Source: CAD feature listing. Evaluate the final solid. Frame: model axes, mm. A direction names the side the tool comes from. Coordinates: 2 decimals unless noted, no trailing zeros. Loops run counter-clockwise (first coordinate to the right, second up) from the corner with the lowest first, then second, coordinate; pieces in that order, holes last. Notation, with made-up numbers: M -13.5,10 L 36.5,10 A16 cw 36.5,17 Z; hole C -0.5,-31 d4. An arc over 180 degrees is marked long. One line per question, with ' | ' between items. Start each with the question number.
1. Access query for faces 4 (the flat face through (1, 20, -46)), 5 (the flat face through (36, -3, -5)), 6 (the flat face through (2, 11, -47)). Directions: +Z, -Z, +X, -X, +Y, -Y. A direction counts if a zero-diameter tool reaches every point of the face in a straight line with its end or side. Return the directions, or none.
2. Section query D-D, the plane y = -1. Output: boundary loops of the cut face in (x, z), and give its area (3 significant figures).
3. Ray query, probe 1 along Z at (x, y) = (68, 11.75); probe 2 along Z at (x, y) = (6, 5); probe 3 along X at (y, z) = (14, -62). Return the intervals inside material, ascending.
4. Section query C-C, the plane z = -58. Output: boundary loops of the cut face in (x, y), and give its area (3 significant figures).
5. Mould query, pull axis Z, two halves, no side actions, for faces 1 (the flat face through (37, 2, -47)), 2 (the flat face through (36, -7, -89)), 3 (the flat face through (37, 7, 0)). Classes: pulls with the +Z half, pulls with the -Z half, needs draft (parallel to the pull), parting line crosses it, or undercut.
6. Pin query (flat end, axial travel): P1, Ø6, axis at x = 48, z = -40, coming from the +Y side; P2, Ø10, axis at x = 16, z = -67, coming from the -Y side. Return the tip coordinate at first contact, or that it passes through.
7. Section query B-B, the plane x = 65.5. Output: boundary loops of the cut face in (y, z), and give its area (3 significant figures).
```python
from build123d import *

# Parameters (mm, degrees)
SKETCH_1_W          = 74
SKETCH_1_H          = 65
EXTRUDE_1_DEPTH     = 20
SKETCH_2_W          = 70
SKETCH_2_H          = 61
CUT_EXTRUDE_1_DEPTH = 18
SKETCH_3_W          = 5
SKETCH_3_H          = 2
CUT_EXTRUDE_2_DEPTH = 18
SKETCH_4_W          = 74
SKETCH_4_H          = 27
EXTRUDE_2_DEPTH     = 20
CUT_EXTRUDE_3_DEPTH = 18
SKETCH_6_W          = 74
SKETCH_6_H          = 5
EXTRUDE_3_DEPTH     = 7
FILLET_1_R          = 2
FILLET_2_R          = 2
FILLET_3_R          = 2
FILLET_5_R          = 1


with BuildPart() as part:
    # 草图1 → 凸台-拉伸1 (new body)
    with BuildSketch(Plane(origin=(0, 0, 0), x_dir=(1, 0, 0), z_dir=(0, 1, 0))):
        with Locations((37, 32.5)):
            Rectangle(SKETCH_1_W, SKETCH_1_H)
    extrude(amount=EXTRUDE_1_DEPTH)

    # 草图2 → 切除-拉伸1 (cut)
    with BuildSketch(Plane(origin=(0, 20, 0), x_dir=(1, 0, 0), z_dir=(0, 1, 0))):
        with Locations((37, 32.5)):
            Rectangle(SKETCH_2_W, SKETCH_2_H)
    extrude(amount=-CUT_EXTRUDE_1_DEPTH, mode=Mode.SUBTRACT)

    # 草图3 → 切除-拉伸2 (cut)
    with BuildSketch(Plane(origin=(0, 20, 0), x_dir=(1, 0, 0), z_dir=(0, 1, 0))):
        with Locations((4.5, 64)):
            Rectangle(SKETCH_3_W, SKETCH_3_H)
    extrude(amount=-CUT_EXTRUDE_2_DEPTH, mode=Mode.SUBTRACT)

    # 草图4 → 凸台-拉伸2 (add)
    with BuildSketch(Plane.XZ):
        with Locations((37, -78.5)):
            Rectangle(SKETCH_4_W, SKETCH_4_H)
    extrude(amount=-EXTRUDE_2_DEPTH)

    # 草图5 → 切除-拉伸3 (cut)
    with BuildSketch(Plane(origin=(0, 20, 0), x_dir=(1, 0, 0), z_dir=(0, 1, 0))):
        Polygon((2, 65), (7, 65), (72, 65), (72, 90), (2, 90), align=None)
    extrude(amount=-CUT_EXTRUDE_3_DEPTH, mode=Mode.SUBTRACT)

    # 草图6 → 凸台-拉伸3 (add)
    with BuildSketch(Plane.XZ):
        with Locations((37, -2.5)):
            Rectangle(SKETCH_6_W, SKETCH_6_H)
        with Locations((37, -89.5)):
            Rectangle(SKETCH_6_W, SKETCH_6_H)
    extrude(amount=EXTRUDE_3_DEPTH)

    # 圆角1
    fillet_1_edges = [part.edges().sort_by_distance(p)[0] for p in [
        (0, 6.5, 0),
    ]]
    fillet(fillet_1_edges, radius=FILLET_1_R)

    # 圆角2
    fillet_2_edges = [part.edges().sort_by_distance(p)[0] for p in [
        (74, 6.5, 0),
    ]]
    fillet(fillet_2_edges, radius=FILLET_2_R)

    # 圆角3
    fillet_3_edges = [part.edges().sort_by_distance(p)[0] for p in [
        (0, 6.5, -92),
        (74, 6.5, -92),
    ]]
    fillet(fillet_3_edges, radius=FILLET_3_R)

    # 圆角5
    fillet_5_edges = [part.edges().sort_by_distance(p)[0] for p in [
        (7, 11, -65),
        (7, 11, -63),
    ]]
    fillet(fillet_5_edges, radius=FILLET_5_R - 0.0001)  # a hair under: the kernel refuses the full size


solid = part.part
```
Taken from the geometry:
1) face 4: +Z, -Z, +X, -X, +Y | face 5: +X, -X, -Y | face 6: +Y
2) outline: M 0,-90 A2 ccw 2,-92 L 72,-92 A2 ccw 74,-90 L 74,-87 L 0,-87 Z; M 0,-5 L 74,-5 L 74,-2 A2 ccw 72,0 L 2,0 A2 ccw 0,-2 Z | area: 737 mm^2
3) probe 1: -92 to -90, -65 to -63, -2 to 0 | probe 2: -92 to -90, -2 to 0 | probe 3: 0 to 2, 72 to 74
4) outline: M 0,0 L 74,0 L 74,20 L 72,20 L 72,2 L 2,2 L 2,20 L 0,20 Z | area: 220 mm^2
5) face 1: undercut | face 2: needs draft | face 3: pulls with the +Z half
6) P1: y = 2 | P2: y = 0
7) outline: M -7,-92 L 20,-92 L 20,-90 L 2,-90 L 2,-65 L 20,-65 L 20,-63 L 2,-63 L 2,-2 L 20,-2 L 20,0 L -7,0 L -7,-5 L 0,-5 L 0,-87 L -7,-87 Z | area: 362 mm^2
